Geometry: final body of the model. Coordinates: model frame, mm. A direction names the side the tool comes from. Round coordinates to 2 decimals unless told otherwise and drop trailing zeros. Loops run counter-clockwise (first coordinate to the right, second up) from the corner with the lowest first, then second, coordinate; pieces in that order, holes last. Notation, with made-up numbers: (-23.75, 69.25) - (-4.75, 69.25) arc R14 ccw to (-4.75, 96.25) - close; hole circle Ø10 at (-4.75, 82). An arc over 180 degrees is marked (long way). Write item = value, one per line. Start each with the question number.
Item 1: Draft query along Y for faces 1 (the flat face through (-5, -6.35, -11)), 2 (the flat face through (-16, -3, -6.677)), 3 (the cylindrical face through (-16.5, -4, -14.2)). Return one class per face: pulls with the +Y half, pulls with the -Y half, needs draft (parallel to the pull), parting line crosses it, or undercut.
Item 2: Access query for faces 4 (the flat face through (-21, -3, -1.68)), 5 (the flat face through (20, -3, -1.68)), 6 (the cylindrical face through (-16.5, -4, -3.1)), 7 (the flat face through (-16, -3, -5.089)), 8 (the cylindrical face through (-13.2, -3.1, -14.8)). Directions: +Z, -Z, +X, -X, +Y, -Y. A direction counts if a zero-diameter tool reaches every point of the face in a straight line with its end or side. Return the directions, or none.
Item 3: First-contact query: pin 1 (3 mm diameter, centred on x = -20, y = -2, fed in from +Z); pin 2 (1 mm diameter, centred on y = -5, z = 1, fed in from +X); pin 3 (21.5 mm diameter, centred on x = 0, z = 0, fed in from +Y). Flat tips, straight axial feed; report the tip coordinate or a pass-through.
Item 4: Section B-B (x = 12.7). Return loops of the section in (y, z), plus the area to 3 significant figures.
Item 5: Section D-D (x = -12.7). Return loops of the section in (y, z), plus the area to 3 significant figures.
Item 6: Section A-A (z = -12.7). Return loops of the section in (x, y) (3 decimals), plus the area to 3 significant figures.
Item 7: Section C-C (z = -4). Return loops of the section in (x, y) (3 decimals), plus the area to 3 significant figures.
Item 8: Line query: line 1 (X direction, y = -1.5, z = -3); line 2 (Y direction, x = -18.5, z = -18); line 3 (Z direction, x = -13, y = -3.25). Output: solid intervals per line, ascending. Write a range as from..to.
from build123d import *

# Parameters (mm, degrees)
F0_R     = 2.159
F1_DEPTH = 6.35
F2_R     = 2.159
F3_DEPTH = 38.1


with BuildPart() as f1:
    # F0 (on Front) → F1 (new body)
    with BuildSketch(Plane.XZ):
        with BuildLine():
            ThreePointArc((-10.70052, -5.089209), (10.275417, 5.90059), (-9.788908, -6.676709))
            Line((-9.788908, -6.676709), (-21.670413, -6.676709))
            Line((-21.670413, -6.676709), (-21.670413, -22.018309))
            Line((-21.670413, -22.018309), (21.670413, -22.018309))
            Line((21.670413, -22.018309), (21.670413, -1.679891))
            Line((21.670413, -1.679891), (18.137582, -1.679891))
            ThreePointArc((18.137582, -1.679891), (15.986714, -0.840354), (14.973315, 1.234274))
            ThreePointArc((14.973315, 1.234274), (0, 15.0241), (-14.973315, 1.234274))
            ThreePointArc((-14.973315, 1.234274), (-15.986714, -0.840354), (-18.137582, -1.679891))
            Line((-18.137582, -1.679891), (-21.670413, -1.679891))
            Line((-21.670413, -1.679891), (-21.670413, -5.089209))
            Line((-21.670413, -5.089209), (-10.70052, -5.089209))
        make_face()
        with Locations((-12.7, -12.7)):
            Circle(F0_R, mode=Mode.SUBTRACT)
        with Locations((12.7, -12.7)):
            Circle(F0_R, mode=Mode.SUBTRACT)
    extrude(amount=F1_DEPTH)

    # F2 (on face) → F3 (cut, symmetric)
    with BuildSketch(Plane.XY.offset(-1.679891)):
        with Locations((-18.495413, -3.175)):
            Circle(F2_R)
    extrude(amount=F3_DEPTH, both=True, mode=Mode.SUBTRACT)


solid = f1.part
Taken from the geometry:
q1.face_1 = pulls with the -Y half
q1.face_2 = needs draft
q1.face_3 = undercut
q2.face_4 = +Z, -X, +Y, -Y
q2.face_5 = +Z, +X, +Y, -Y
q2.face_6 = +Z, -Z
q2.face_7 = -X, +Y, -Y
q2.face_8 = +Y, -Y
q3.pin_1 = -1.68
q3.pin_2 = 15.12
q3.pin_3 = through
q4.outline = (-6.35, -22.02) - (0, -22.02) - (0, -14.86) - (-6.35, -14.86) - close; (-6.35, -10.54) - (0, -10.54) - (0, 8.03) - (-6.35, 8.03) - close
q4.area = 163 mm^2
q5.outline = (-6.35, -22.02) - (0, -22.02) - (0, -14.86) - (-6.35, -14.86) - close; (-6.35, -10.54) - (0, -10.54) - (0, -6.68) - (-6.35, -6.68) - close; (-6.35, -5.09) - (0, -5.09) - (0, 8.03) - (-6.35, 8.03) - close
q5.area = 153 mm^2
q6.outline = (-21.67, -6.35) - (-14.859, -6.35) - (-14.859, 0) - (-21.67, 0) - close; (-10.541, -6.35) - (10.541, -6.35) - (10.541, 0) - (-10.541, 0) - close; (14.859, -6.35) - (21.67, -6.35) - (21.67, 0) - (14.859, 0) - close; hole circle Ø4.318 at (-18.495, -3.175)
q6.area = 206 mm^2
q7.outline = (-21.67, -6.35) - (-11.154, -6.35) - (-11.154, 0) - (-21.67, 0) - close; (11.154, -6.35) - (21.67, -6.35) - (21.67, 0) - (11.154, 0) - close; hole circle Ø4.318 at (-18.495, -3.175)
q7.area = 119 mm^2
q8.line_1 = -21.67..-19.86, -17.13..-11.46, 11.46..21.67
q8.line_2 = -6.35..-5.33, -1.02..0
q8.line_3 = -22.02..-14.84, -10.56..-6.68, -5.09..7.53
